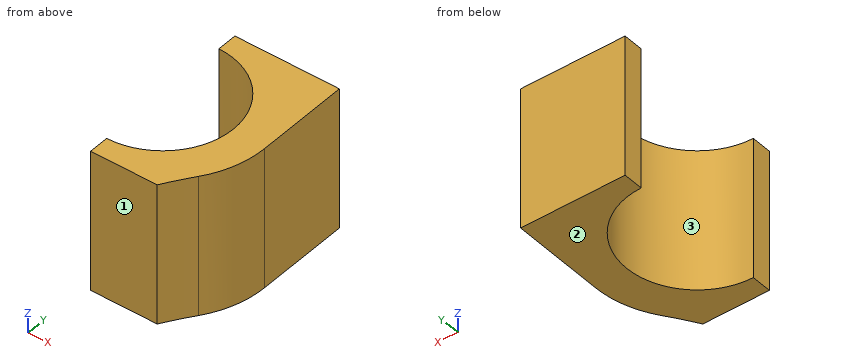
```python
from build123d import *

# Parameters (mm, degrees)
EXTRUDE_1_DEPTH = 14


with BuildPart() as part:
    # 草图1 → 凸台-拉伸1 (new body)
    with BuildSketch(Plane.XY):
        with BuildLine():
            Line((-4.335050742, 439.946209227), (-4.335050742, 449.276757584))
            Line((-4.335050742, 449.276757584), (-14.712951443, 449.276757584))
            Line((-14.712951443, 449.276757584), (-14.712951443, 447.276757584))
            ThreePointArc((-14.712951443, 447.276757584), (-7.712951443, 440.276757584), (-14.712951443, 433.276757584))
            Line((-14.712951443, 433.276757584), (-14.712951443, 431.276757584))
            Line((-14.712951443, 431.276757584), (-8.105031432, 431.276757584))
            ThreePointArc((-8.105031432, 431.276757584), (-7.200115769, 432.694505685), (-6.239812646, 434.075338748))
            ThreePointArc((-6.239812646, 434.075338748), (-4.823153429, 436.860142228), (-4.335050742, 439.946209227))
        make_face()
    extrude(amount=EXTRUDE_1_DEPTH)


solid = part.part
```
For this review, take the finished solid that the model builds, in its own axes (mm). Face numbers are marked on the shaded views. Coordinates: 2 decimals unless noted, no trailing zeros. Loops run counter-clockwise (first coordinate to the right, second up) from the corner with the lowest first, then second, coordinate; pieces in that order, holes last.
1. Insertion check: P1, Ø4, axis at x = -12, y = 444, coming from the +Z side; P2, Ø1, axis at y = 440.5, z = 12, coming from the -X side. Each pin has a flat end and moves straight along its axis. Give the tip position at first contact, or say it passes through.
2. Add section C-C, the plane x = -14. Give the boundary of the cut face in (y, z), then the cut area to 3 significant figures.
3. Mouldability with a two-part tool opening along Y and no side actions: class the marked faces 1, 2 and 3 as +Y half, -Y half, draft (parallel to the pull), parting line (faces both ways), or undercut.
4. Add section A-A, the plane x = -10.5. Give the boundary of the cut face in (y, z).
5. Add section D-D, the plane y = 446.25. Give the boundary of the cut face in (x, z), then the cut area to 3 significant figures.
6. For line 1 (Y direction, x = -12.5, z = 4); line 2 (Y direction, x = -11.5, z = 5.75); line 3 (X direction, y = 442, z = 9.5), list the stretches that pass through material, from the lowest coordinate up.
7. Add section B-B, the plane z = 8. Give the boundary of the cut face in (x, y).
Result:
1. P1: passes through
1. P2: stops at x = -7.75
2. outline: (431.28, 0) - (433.31, 0) - (433.31, 14) - (431.28, 14) - close; (447.24, 0) - (449.28, 0) - (449.28, 14) - (447.24, 14) - close
2. area: 57.0 mm2
3. face 1: -Y half
3. face 2: draft
3. face 3: undercut
4. outline: (431.28, 0) - (434.69, 0) - (434.69, 14) - (431.28, 14) - close; (445.87, 0) - (449.28, 0) - (449.28, 14) - (445.87, 14) - close
5. outline: (-11.06, 0) - (-4.34, 0) - (-4.34, 14) - (-11.06, 14) - close
5. area: 94.2 mm2
6. line 1: y = 431.28 to 433.64, 446.92 to 449.28
6. line 2: y = 431.28 to 434.06, 446.5 to 449.28
6. line 3: x = -7.93 to -4.34
7. outline: (-14.71, 431.28) - (-8.11, 431.28) arc R42.5 cw to (-6.24, 434.08) arc R10 ccw to (-4.34, 439.95) - (-4.34, 449.28) - (-14.71, 449.28) - (-14.71, 447.28) arc R7 cw to (-14.71, 433.28) - close
